For this review, take the finished solid that the model builds, in its own axes (mm). Face numbers are marked on the shaded views. A direction names the side the tool comes from. Round coordinates to 2 decimals unless told otherwise and drop trailing zeros. Loops run counter-clockwise (first coordinate to the right, second up) from the corner with the lowest first, then second, coordinate; pieces in that order, holes last. Notation, with made-up numbers: (15, -37.5) -> (26, -37.5) arc R21 cw to (26, -11.5) -> close; hole circle Ø3 at (76.5, -27.75). An arc over 180 degrees is marked (long way). Write each question's results on one line, items separated by ' | '.
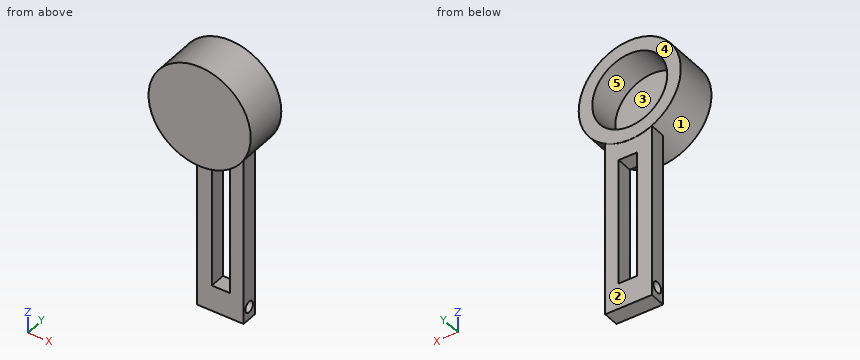
```python
from build123d import *

# Parameters (mm, degrees)
F0_R      = 29.3755194238
F0_R_2    = 20.4584720474
F1_DEPTH  = 25.4
F3_W      = 26.813134551
F3_H      = 9.2550148256
F4_DEPTH  = 102.5347784162
F2_R      = 21.5684000446
F5_DEPTH  = 19.05
F7_R      = 3.175
F8_DEPTH  = 50.8
F9_W      = 10.5024166405
F9_H      = 73.061581701
F10_DEPTH = 25.4


with BuildPart() as f1:
    # F0 (on Front) → F1 (new body)
    with BuildSketch(Plane.XZ):
        with Locations((-56.8432807922, 24.0650400519)):
            Circle(F0_R)
        with Locations((-56.8432807922, 24.0650400519)):
            Circle(F0_R_2, mode=Mode.SUBTRACT)
        with Locations((-56.8432807922, 24.0650400519)):
            Circle(F0_R_2)
    extrude(amount=F1_DEPTH)

    # F3 (on Top) → F4 (join)
    with BuildSketch(Plane.XY):
        with Locations((-56.0491830111, -4.7410854604)):
            Rectangle(F3_W, F3_H)
    extrude(amount=-F4_DEPTH)

    # F2 (on face) → F5 (cut)
    with BuildSketch(Plane(origin=(0, 0, 0), x_dir=(-1, 0, 0), z_dir=(0, 1, 0))):
        with Locations((56.8432807922, 24.0650400519)):
            Circle(F2_R)
    extrude(amount=-F5_DEPTH, mode=Mode.SUBTRACT)

    # F7 (on face) → F8 (cut)
    with BuildSketch(Plane.YZ.offset(-42.6426157355)):
        with Locations((-4.7467201948, -95.2464714646)):
            Circle(F7_R)
    extrude(amount=-F8_DEPTH, mode=Mode.SUBTRACT)

    # F9 (on face) → F10 (cut)
    with BuildSketch(Plane(origin=(0, -0.1135780476, 0), x_dir=(-1, 0, 0), z_dir=(0, 1, 0))):
        with Locations((55.6544419378, -51.0808248073)):
            Rectangle(F9_W, F9_H)
    extrude(amount=-F10_DEPTH, mode=Mode.SUBTRACT)


solid = f1.part
```
1. For pin 1 (10 mm diameter, centred on y = -5, z = 32.5, fed in from +X); pin 2 (4.5 mm diameter, centred on y = -5.5, z = -40, fed in from +X); pin 3 (1 mm diameter, centred on x = -39, y = -4.5, fed in from +Z); pin 4 (12 mm diameter, centred on y = -15.5, z = -74, fed in from +X), all flat-tipped, find the tip position at first contact; note any pin that passes through.
Values found:
pin 1: stops at x = -27.67 | pin 2: stops at x = -42.64 | pin 3: stops at z = 47.77 | pin 4: passes through
2. Consider section B-B (x = -56.5). State the section outline as (y, z) points (3 decimals).
Values found:
outline: (-25.4, -5.308) -> (-9.369, -5.308) -> (-9.369, -14.55) -> (-0.114, -14.55) -> (-0.114, -5.308) -> (0, -5.308) -> (0, 2.499) -> (-19.05, 2.499) -> (-19.05, 45.631) -> (0, 45.631) -> (0, 53.439) -> (-25.4, 53.439) -> close; (-9.369, -102.535) -> (-0.114, -102.535) -> (-0.114, -87.612) -> (-9.369, -87.612) -> close; hole circle Ø6.35 at (-4.747, -95.246)
3. Draft analysis for pull direction Z (two halves, no side actions). For the marked faces 1, 2 and 3, state which applies: released by +Z, released by -Z, zero draft, split by the parting line, or undercut.
Values found:
face 1: split by the parting line | face 2: zero draft | face 3: undercut
4. To check wall thickness, follow probe 1 along X at (y, z) = (-6.75, -84); probe 2 along Z at (x, y) = (-66, -2.75); probe 3 along Z at (x, y) = (-44, -3.25). State the ranges of each line that lie inside material, in increasing order.
Values found:
probe 1: x = -69.46 to -60.91, -50.4 to -42.64 | probe 2: z = -102.53 to -97.72, -92.78 to 4.54, 43.59 to 51.98 | probe 3: z = -102.53 to -98.05, -92.45 to 6.74, 41.39 to 50.48
5. Consider section C-C (y = -4.5). State the section outline as (x, z) points.
Values found:
outline: (-69.46, -102.53) -> (-42.64, -102.53) -> (-42.64, -98.41) -> (-69.46, -98.41) -> close; (-69.46, -92.08) -> (-42.64, -92.08) -> (-42.64, -1.65) arc R29.38 ccw (long way) to (-69.46, -2.47) -> close; hole circle Ø43.14 at (-56.84, 24.07); hole (-60.91, -87.61) -> (-50.4, -87.61) -> (-50.4, -14.55) -> (-60.91, -14.55) -> close
6. Tool access review of the marked faces 4 and 5: name each direction out of +Z, -Z, +X, -X, +Y, -Y from which nothing blocks a thin tool from reaching the whole face with its end or side.
Values found:
face 4: +Z, -Z, +X, -X, +Y | face 5: +Y
7. Consider section A-A (z = -81). State the section outline as (x, y) points, plus the area to 3 significant figures.
Values found:
outline: (-69.46, -9.37) -> (-60.91, -9.37) -> (-60.91, -0.11) -> (-69.46, -0.11) -> close; (-50.4, -9.37) -> (-42.64, -9.37) -> (-42.64, -0.11) -> (-50.4, -0.11) -> close | area: 151 mm2
